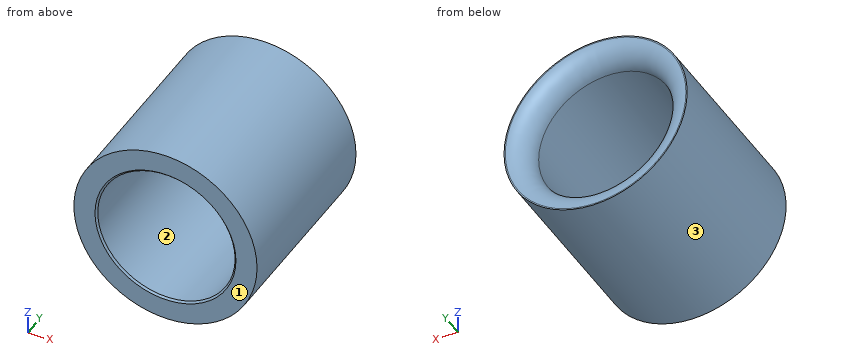
```python
from build123d import *

# Parameters (mm, degrees)
F0_R     = 50.8
F0_R_2   = 38.1
F1_DEPTH = 101.2
F2_R     = 12
F3_SIZE  = 1


with BuildPart() as f1:
    # F0 (on Front) → F1 (new body)
    with BuildSketch(Plane.XZ):
        Circle(F0_R)
        Circle(F0_R_2, mode=Mode.SUBTRACT)
    extrude(amount=F1_DEPTH)

    # F2
    f2_edges = [f1.edges().sort_by_distance(p)[0] for p in [
        (-38.1, 0, 0),
    ]]
    fillet(f2_edges, radius=F2_R)

    # F3
    f3_edges = [f1.edges().sort_by_distance(p)[0] for p in [
        (38.1, -56.6, 0),
        (-38.1, -12, 0),
        (-38.1, -101.2, 0),
    ]]
    chamfer(f3_edges, length=F3_SIZE)


solid = f1.part
```
Input: part model. Units: mm. Frame: model coordinates. Face numbers are marked on the shaded views. Coordinates: 2 decimals unless noted, no trailing zeros. Loops run counter-clockwise (first coordinate to the right, second up) from the corner with the lowest first, then second, coordinate; pieces in that order, holes last. Notation, with made-up numbers: M -19.5,-28.5 L 14.5,-28.5 A20 cw 14.5,1.5 Z; hole C 66.5,11.25 d11. An arc over 180 degrees is marked long. One line per item, written item: value.
(1) Section D-D (y = -9). Output: boundary loops of the cut face in (x, z), and give its area (3 significant figures).
Filled in:
outline: C 0,0 d101.6; hole C 0,0 d76.96
area: 3,460 mm^2
(2) Line query: line 1 along Z through (x, y) = (0, -51); line 2 along X through (y, z) = (-54.5, 24); line 3 along X through (y, z) = (-53, -16.5). Output: solid intervals per line, ascending. Write a range as from..to.
Filled in:
line 1: -50.8..-38.1, 38.1..50.8
line 2: -44.77..-29.59, 29.59..44.77
line 3: -48.05..-34.34, 34.34..48.05
(3) Pull-direction query (X, two-part tool) for the marked faces 1, 2 and 3; classes: +X half, -X half, draft (parallel to the pull), parting line (faces both ways), or undercut.
Filled in:
face 1: draft
face 2: undercut
face 3: parting line
(4) Section B-B (z = 0). Output: boundary loops of the cut face in (x, y).
Filled in:
outline: M -50.8,-101.2 L -39.1,-101.2 L -38.1,-100.2 L -38.1,-12 A12 ccw -50.1,0 L -50.8,0 Z; M 38.1,-100.2 L 39.1,-101.2 L 50.8,-101.2 L 50.8,0 L 50.1,0 A12 ccw 38.1,-12 Z
(5) Pin query (flat end, axial travel): pin 1 (1.5 mm diameter, centred on x = 23.5, y = -69.5, fed in from -Z); pin 2 (2 mm diameter, centred on x = 0, y = -31, fed in from -Z); pin 3 (12 mm diameter, centred on x = 19, z = 32, fed in from +Y). Return the tip coordinate at first contact, or that it passes through.
Filled in:
pin 1: z = -45.42
pin 2: z = -50.8
pin 3: y = -2.17
(6) Section A-A (x = 0). Output: boundary loops of the cut face in (y, z), and give its area (3 significant figures).
Filled in:
outline: M -101.2,-50.8 L 0,-50.8 L 0,-50.1 A12 ccw -12,-38.1 L -100.2,-38.1 L -101.2,-39.1 Z; M -101.2,39.1 L -100.2,38.1 L -12,38.1 A12 ccw 0,50.1 L 0,50.8 L -101.2,50.8 Z
area: 2,510 mm^2
(7) Section C-C (y = -93.5). Output: boundary loops of the cut face in (x, z).
Filled in:
outline: C 0,0 d101.6; hole C 0,0 d76.2
